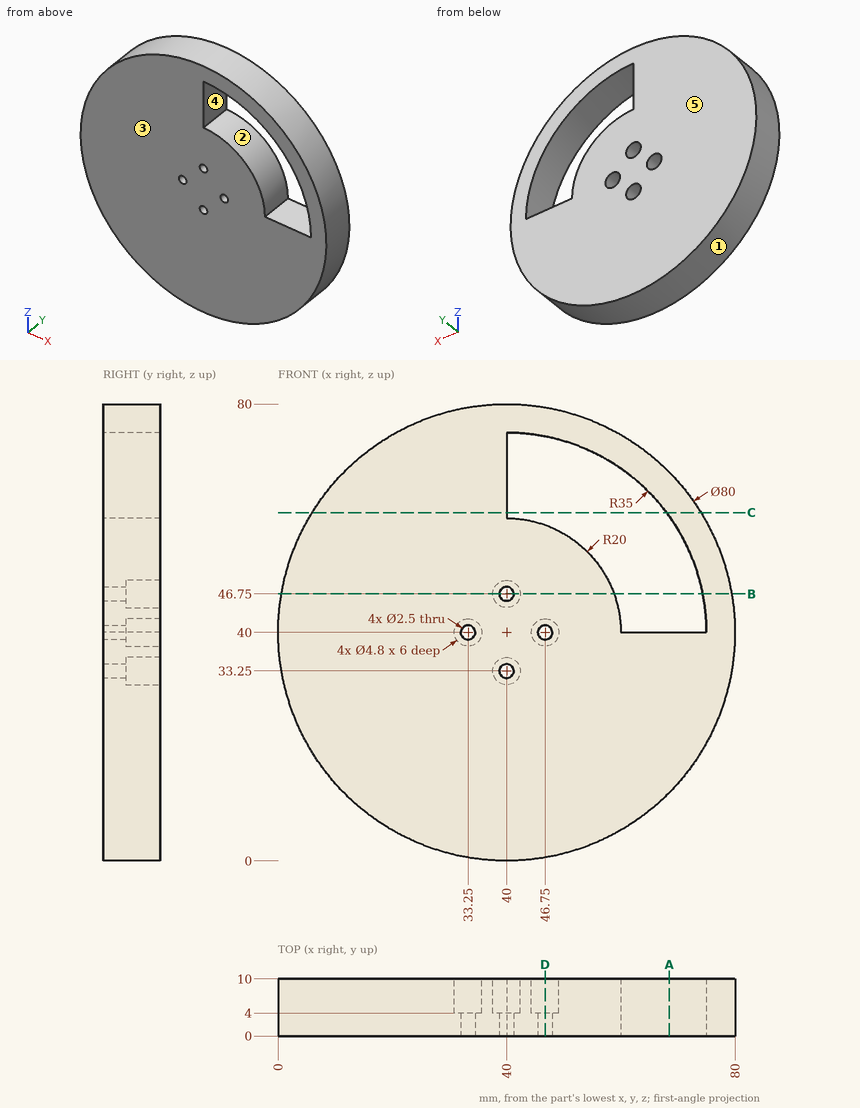
Geometry: see drawing. Coordinates: mm, zero at the bounding-box minimum. A direction names the side the tool comes from. Coordinates: 2 decimals unless noted, no trailing zeros. Order: outer loops, then holes, each group sorted by start corner. A loop starts at its lowest first (then second) coordinate and runs counter-clockwise, first axis right, second up. Notation, with made-up numbers: (6, 72.25) - (55, 72.25) arc R17 cw to (55, 78.25) - close; hole circle Ø6 at (-34, 10.5). An arc over 180 degrees is marked (long way). Use one line per item in the form item = value.
1) Section A-A (x = 68.5). Return loops of the section in (y, z), then the cut area to 3 significant figures.
Solutions:
outline = (0, 11.93) - (10, 11.93) - (10, 40) - (0, 40) - close; (0, 60.32) - (10, 60.32) - (10, 68.07) - (0, 68.07) - close
area = 358 mm^2
2) Section B-B (z = 46.75). Return loops of the section in (x, y), then the cut area to 3 significant figures.
Solutions:
outline = (0.57, 0) - (38.75, 0) - (38.75, 4) - (37.6, 4) - (37.6, 10) - (0.57, 10) - close; (41.25, 0) - (58.83, 0) - (58.83, 10) - (42.4, 10) - (42.4, 4) - (41.25, 4) - close; (74.34, 0) - (79.43, 0) - (79.43, 10) - (74.34, 10) - close
area = 595 mm^2
3) Pin query (flat end, axial travel): pin 1 (2.5 mm diameter, centred on x = 40.5, z = 46, fed in from +Y); pin 2 (2 mm diameter, centred on x = 46.75, z = 40, fed in from -Y); pin 3 (3 mm diameter, centred on y = 5.5, z = 48, fed in from +X); pin 4 (2 mm diameter, centred on x = 53.5, y = 7, fed in from -Z). Return the tip coordinate at first contact, or that it passes through.
Solutions:
pin_1 = 4
pin_2 = through
pin_3 = 79.47
pin_4 = 2
4) Mould query, pull axis X, two halves, no side actions, for the marked faces 1, 2 and 3. Classes: +X half, -X half, draft (parallel to the pull), parting line (faces both ways), or undercut.
Solutions:
face_1 = parting line
face_2 = undercut
face_3 = draft
5) Section C-C (z = 61). Return loops of the section in (x, y).
Solutions:
outline = (5.96, 0) - (40, 0) - (40, 10) - (5.96, 10) - close; (68, 0) - (74.04, 0) - (74.04, 10) - (68, 10) - close
6) Ray query, L1, parallel to Z at x = 47.5, y = 3.75; L2, parallel to X at y = 2.65, z = 46.75; L3, parallel to Z at x = 70, y = 7.75. Return the intervals inside material, ascending.
Solutions:
L1 = 0.71 to 39, 41 to 58.54, 74.19 to 79.29
L2 = 0.57 to 38.75, 41.25 to 58.83, 74.34 to 79.43
L3 = 13.54 to 40, 58.03 to 66.46
7) Set-up query: the marked faces 4 and 5. Return all of +Z, -Z, +X, -X, +Y, -Y with unobstructed straight access to the full face (end or side cutting, diameter ignored); none if empty.
Solutions:
face_4 = +Y, -Y
face_5 = +Z, -Z, +X, -X, +Y
8) Section D-D (x = 46.75). Return loops of the section in (y, z), then the cut area to 3 significant figures.
Solutions:
outline = (0, 0.57) - (10, 0.57) - (10, 37.6) - (4, 37.6) - (4, 38.75) - (0, 38.75) - close; (0, 41.25) - (4, 41.25) - (4, 42.4) - (10, 42.4) - (10, 58.83) - (0, 58.83) - close; (0, 74.34) - (10, 74.34) - (10, 79.43) - (0, 79.43) - close
area = 595 mm^2
